Could you check a few things on this model? Use its own coordinates, in mm. Give positions to 0.01 mm unless a question says otherwise; leave off trailing zeros. Loops run counter-clockwise (first coordinate to the right, second up) from the corner with the lowest first, then second, coordinate; pieces in that order, holes last. Notation, with made-up numbers: (20, 53) - (34, 53) arc R22 cw to (34, 79) - close; hole circle Ø10 at (57.25, -26). An arc over 180 degrees is marked (long way). Write each question's results on one line, items separated by ' | '. Start each with the question number.
1) I'm going to push flat-ended pins straight in: pin 1 (1.5 mm diameter, centred on x = -14, y = 4.5, fed in from -Z); pin 2 (5 mm diameter, centred on y = -3, z = 4.5, fed in from -X); pin 3 (6 mm diameter, centred on x = 47.5, y = 4.5, fed in from -Z); pin 4 (18 mm diameter, centred on x = 0, z = -110, fed in from -Y). Where does each tip first touch, or does it pass through?
2) I want a section at C-C, the plane y = 2.25. Write out the boundary of the cut face in (x, z), and give its area (3 significant figures).
3) I want a section at A-A, the plane z = 52. Write out the boundary of the cut face in (x, y).
4) If I drill on probe 1 along X at (y, z) = (2.5, 52); probe 2 along X at (y, z) = (4.5, -13.5); probe 3 along X at (y, z) = (3.75, -111), over which ranges is the centre line in solid material (lowest first)? Write a range as [from, to].
5) I want a section at B-B, the plane x = 0. Write out the boundary of the cut face in (y, z), and give its area (3 significant figures).
6) I want a section at D-D, the plane z = -110. Write out the boundary of the cut face in (x, y), and give its area (3 significant figures).
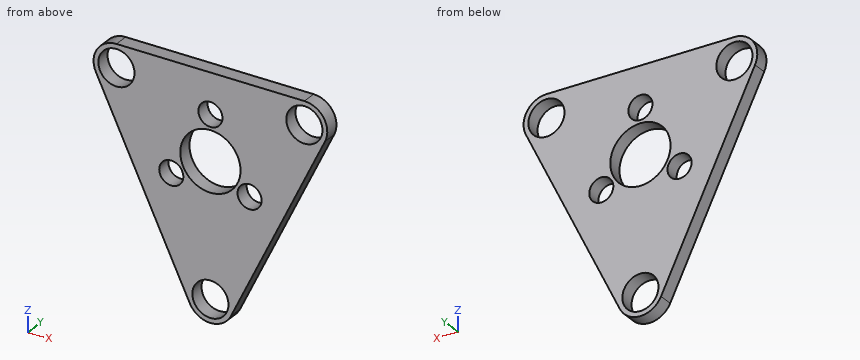
from build123d import *

# Parameters (mm, degrees)
SKETCH1_R           = 15
SKETCH1_R_2         = 25
BOSS_EXTRUDE1_DEPTH = 6
HOLE1_D             = 20
CIRPATTERN1_COUNT   = 3


with BuildPart() as part:
    # Sketch1 → Boss-Extrude1 (new, symmetric)
    with BuildSketch(Plane(origin=(0, 0, 0), x_dir=(1, 0, 0), z_dir=(0, 1, 0))):
        with BuildLine():
            Line((-95.119031725, -43.757503243), (-17.119031725, 118.242496757))
            ThreePointArc((-17.119031725, 118.242496757), (0, 129), (17.119031725, 118.242496757))
            Line((17.119031725, 118.242496757), (95.119031725, -43.757503243))
            ThreePointArc((95.119031725, -43.757503243), (94.087377636, -62.109217616), (78, -71))
            Line((78, -71), (-78, -71))
            ThreePointArc((-78, -71), (-94.087377636, -62.109217616), (-95.119031725, -43.757503243))
        make_face()
        with Locations(Location((0, 110, 0), (0, 0, 270))):
            Circle(SKETCH1_R, mode=Mode.SUBTRACT)
        with Locations(Location((-78, -52, 0), (0, 0, 270))):
            Circle(SKETCH1_R, mode=Mode.SUBTRACT)
        with Locations(Location((78, -52, 0), (0, 0, 270))):
            Circle(SKETCH1_R, mode=Mode.SUBTRACT)
        with Locations(Location((0, 0, 0), (0, 0, 270))):
            Circle(SKETCH1_R_2, mode=Mode.SUBTRACT)
    extrude(amount=BOSS_EXTRUDE1_DEPTH, both=True)

    # Hole1 (through all)
    with Locations(Plane(origin=(0, 6, 0), x_dir=(1, 0, 0), z_dir=(0, 1, 0))):
        with Locations((0, -37.5)):
            hole1 = Hole(HOLE1_D / 2)

    # CirPattern1: Hole1 ×3 about axis
    cirpattern1_axis = Axis((0, 0, 0), (0, 1, 0))
    for i in range(1, CIRPATTERN1_COUNT):
        add(hole1.rotate(cirpattern1_axis, i * 360 / CIRPATTERN1_COUNT), mode=Mode.SUBTRACT)


solid = part.part
Answers:
1) pin 1: stops at z = -123.62 | pin 2: stops at x = -77.42 | pin 3: stops at z = -61.37 | pin 4: passes through
2) outline: (-95.12, 43.76) - (-17.12, -118.24) arc R19 ccw to (17.12, -118.24) - (95.12, 43.76) arc R19 ccw to (78, 71) - (-78, 71) arc R19 ccw to start; hole circle Ø30 at (-78, 52); hole circle Ø20 at (-32.48, -18.75); hole circle Ø50 at (0, 0); hole circle Ø30 at (0, -110); hole circle Ø20 at (0, 37.5); hole circle Ø20 at (32.48, -18.75); hole circle Ø30 at (78, 52) | area: 18,500 mm2
3) outline: (-97, -6) - (-93, -6) - (-93, 6) - (-97, 6) - close; (-63, -6) - (63, -6) - (63, 6) - (-63, 6) - close; (93, -6) - (97, -6) - (97, 6) - (93, 6) - close
4) probe 1: x = [-97, -93], [-63, 63], [93, 97] | probe 2: x = [-67.55, -40.99], [-23.96, -21.04], [21.04, 23.96], [40.99, 67.55] | probe 3: x = [-20.61, -14.97], [14.97, 20.61]
5) outline: (-6, -129) - (6, -129) - (6, -125) - (-6, -125) - close; (-6, -95) - (6, -95) - (6, -25) - (-6, -25) - close; (-6, 25) - (6, 25) - (6, 27.5) - (-6, 27.5) - close; (-6, 47.5) - (6, 47.5) - (6, 71) - (-6, 71) - close | area: 1,200 mm2
6) outline: (-21.09, -6) - (-15, -6) - (-15, 6) - (-21.09, 6) - close; (15, -6) - (21.09, -6) - (21.09, 6) - (15, 6) - close | area: 146 mm2
